The model under review builds one solid part; all positions refer to its coordinate system, in mm. Coordinates: 2 decimals unless noted, no trailing zeros. Loops run counter-clockwise (first coordinate to the right, second up) from the corner with the lowest first, then second, coordinate; pieces in that order, holes last. Notation, with made-up numbers: (52.25, 72.25) - (109.25, 72.25) arc R14 cw to (109.25, 88.25) - close; hole circle Ø6 at (-9.5, 50). An arc over 180 degrees is marked (long way). One line per item, written item: value. Start each with the question number.
1. We need section B-B, the plane x = -0.75. Give the boundary of the cut face in (y, z), then the cut area to 3 significant figures.
2. To check wall thickness, follow line 1 (X direction, y = 0.85, z = -13.75); line 2 (Z direction, x = 1.25, y = 0.1); line 3 (Z direction, x = 3.5, y = 1.4). State the ranges of each line that lie inside material, in increasing order.
3. We need section C-C, the plane x = 0.5. Give the boundary of the cut face in (y, z), then the cut area to 3 significant figures.
4. Insertion check: P1, Ø1.1, axis at x = 4, z = -9, coming from the -Y side; P2, Ø0.7, axis at x = 2, y = 0.5, coming from the +Z side; P3, Ø1, axis at x = 1.5, z = -11, coming from the -Y side. Each pin has a flat end and moves straight along its axis. Give the tip position at first contact, or say it passes through.
5. We need section A-A, the plane z = -14.25. Give the boundary of the cut face in (x, y), then the cut area to 3 significant figures.
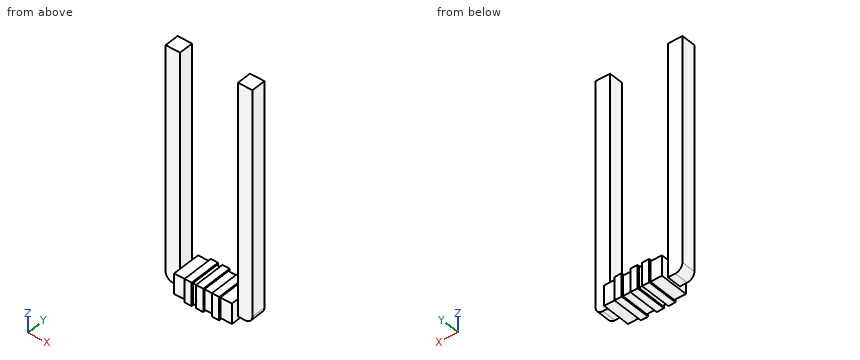
from build123d import *

# Parameters (mm, degrees)
BOSS_EXTRUDE1_DEPTH = 1
SKETCH3_W           = 4
SKETCH3_H           = 1.4
BOSS_EXTRUDE2_DEPTH = 1.5
SKETCH4_W           = 4
SKETCH4_H           = 1.4
CUT_EXTRUDE1_DEPTH  = 1
SKETCH5_W           = 0.5
SKETCH5_H           = 1.6
BOSS_EXTRUDE4_DEPTH = 2.1
SKETCH6_W           = 0.5
SKETCH6_H           = 1.6
BOSS_EXTRUDE5_DEPTH = 0.1


with BuildPart() as part:
    # Sketch1 → Boss-Extrude1 (new body)
    with BuildSketch(Plane(origin=(0, 0, 0), x_dir=(1, 0, 0), z_dir=(0, 1, 0))):
        with BuildLine():
            Line((-1.459627329, 0), (-1.459627329, 15.5))
            ThreePointArc((-1.459627329, 15.5), (-1.31318072, 15.853553391), (-0.959627329, 16))
            Line((-0.959627329, 16), (4.040372671, 16))
            ThreePointArc((4.040372671, 16), (4.393926061, 15.853553391), (4.540372671, 15.5))
            Line((4.540372671, 15.5), (4.540372671, 0))
            Line((4.540372671, 0), (3.540372671, 0))
            Line((3.540372671, 0), (3.540372671, 15))
            Line((3.540372671, 15), (-0.459627329, 15))
            Line((-0.459627329, 15), (-0.459627329, 0))
            Line((-0.459627329, 0), (-1.459627329, 0))
        make_face()
    extrude(amount=BOSS_EXTRUDE1_DEPTH)

    # Sketch3 → Boss-Extrude2 (add, symmetric)
    with BuildSketch(Plane(origin=(0, 1, 0), x_dir=(1, 0, 0), z_dir=(0, 1, 0))):
        with Locations((1.540372671, 15.5)):
            Rectangle(SKETCH3_W, SKETCH3_H)
    extrude(amount=BOSS_EXTRUDE2_DEPTH, both=True)

    # Sketch4 → Cut-Extrude1 (cut)
    with BuildSketch(Plane(origin=(0, 2.5, 0), x_dir=(1, 0, 0), z_dir=(0, 1, 0))):
        with Locations((1.540372671, 15.5)):
            Rectangle(SKETCH4_W, SKETCH4_H)
    extrude(amount=-CUT_EXTRUDE1_DEPTH, mode=Mode.SUBTRACT)

    # Sketch5 → Boss-Extrude4 (add)
    with BuildSketch(Plane(origin=(0, 1.5, 0), x_dir=(1, 0, 0), z_dir=(0, 1, 0))):
        with Locations((0.590372671, 15.5)):
            Rectangle(SKETCH5_W, SKETCH5_H)
        with Locations((1.390372671, 15.5)):
            Rectangle(SKETCH5_W, SKETCH5_H)
        with Locations((2.490372671, 15.5)):
            Rectangle(SKETCH5_W, SKETCH5_H)
    extrude(amount=-BOSS_EXTRUDE4_DEPTH)

    # Sketch6 → Boss-Extrude5 (add)
    with BuildSketch(Plane(origin=(0, 1.5, 0), x_dir=(1, 0, 0), z_dir=(0, 1, 0))):
        with Locations((0.590372671, 15.5)):
            Rectangle(SKETCH6_W, SKETCH6_H)
        with Locations((1.390372671, 15.5)):
            Rectangle(SKETCH6_W, SKETCH6_H)
        with Locations((2.490372671, 15.5)):
            Rectangle(SKETCH6_W, SKETCH6_H)
    extrude(amount=BOSS_EXTRUDE5_DEPTH)


solid = part.part
Findings below:
1. outline: (0, -16) - (1, -16) - (1, 0) - (0, 0) - close
1. area: 16.0 mm2
2. line 1: -1.46 to -0.46, 3.54 to 4.54
2. line 2: -16.3 to -14.7
2. line 3: -16.2 to -14.8
3. outline: (-0.6, -16.3) - (1.6, -16.3) - (1.6, -14.7) - (-0.6, -14.7) - close
3. area: 3.52 mm2
4. P1: y = 0
4. P2: z = -14.7
4. P3: through
5. outline: (-1.46, 0) - (-0.46, 0) - (-0.46, 1) - (-1.46, 1) - close; (3.54, 0) - (4.54, 0) - (4.54, 1) - (3.54, 1) - close
5. area: 2.00 mm2
